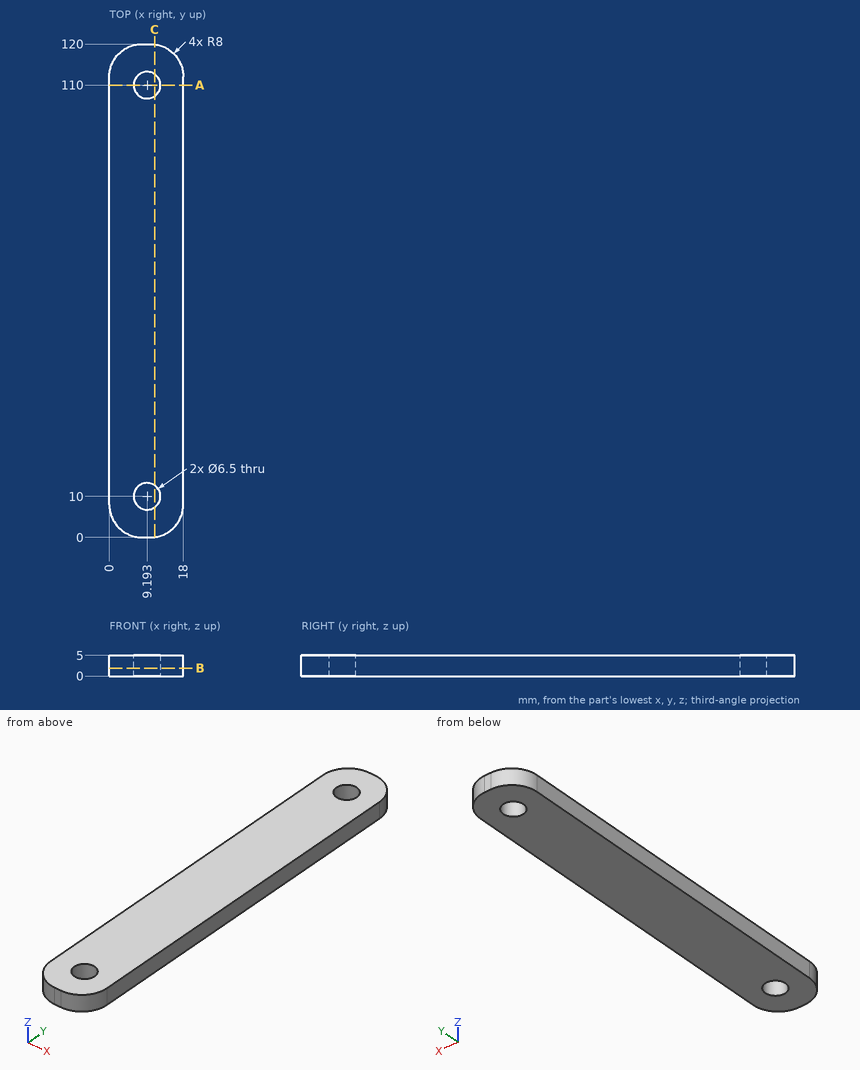
Geometry: see drawing. Coordinates: mm, zero at the bounding-box minimum. Round coordinates to 2 decimals unless told otherwise and drop trailing zeros. Loops run counter-clockwise (first coordinate to the right, second up) from the corner with the lowest first, then second, coordinate; pieces in that order, holes last. Notation, with made-up numbers: (81, 69.5) -> (110, 69.5) arc R20 ccw to (110, 108.5) -> close; hole circle Ø7 at (-24, -25). An arc over 180 degrees is marked (long way). Write each question's results on one line, items separated by ' | '.
1. Ray query, line 1 (Y direction, x = 7, z = 4.1); line 2 (Y direction, x = 9.75, z = 4); line 3 (X direction, y = 7, z = 3.15) (1 decimal). Return the intervals inside material, ascending. Write a range as from..to.
Geometry results:
line 1: 0.06..7.6, 12.4..107.6, 112.4..119.94 | line 2: 0..6.8, 13.2..106.8, 113.2..120 | line 3: 0.1..7.9, 10.4..17.9
2. Section C-C (x = 11). Return loops of the section in (y, z), and give its area (3 significant figures).
Geometry results:
outline: (0.06, 0) -> (7.3, 0) -> (7.3, 5) -> (0.06, 5) -> close; (12.7, 0) -> (107.3, 0) -> (107.3, 5) -> (12.7, 5) -> close; (112.7, 0) -> (119.94, 0) -> (119.94, 5) -> (112.7, 5) -> close | area: 545 mm2
3. Section B-B (z = 1.9). Return loops of the section in (x, y).
Geometry results:
outline: (0, 8) arc R8 ccw to (8, 0) -> (10, 0) arc R8 ccw to (18, 8) -> (18, 112) arc R8 ccw to (10, 120) -> (8, 120) arc R8 ccw to (0, 112) -> close; hole circle Ø6.5 at (9.19, 10); hole circle Ø6.5 at (9.19, 110)
4. First-contact query: P1, Ø1, axis at x = 13.5, z = 2, coming from the +Y side; P2, Ø5, axis at x = 9.19, y = 10, coming from the -Z side. Flat tips, straight axial feed; report the tip coordinate or a pass-through.
Geometry results:
P1: y = 119.42 | P2: through
5. Section A-A (y = 110). Return loops of the section in (x, z), and give its area (3 significant figures).
Geometry results:
outline: (0, 0) -> (5.94, 0) -> (5.94, 5) -> (0, 5) -> close; (12.44, 0) -> (18, 0) -> (18, 5) -> (12.44, 5) -> close | area: 57.5 mm2
